Can you work these out from the model? Positions are in its coordinate system, mm. Give positions to 0.01 mm unless a question says otherwise; leave off trailing zeros.
```python
from build123d import *

# Parameters (mm, degrees)
BOSS_EXTRUDE1_DEPTH = 2
SKETCH2_R           = 1.42
CUT_EXTRUDE2_DEPTH  = 6.35


with BuildPart() as part:
    # Sketch1 → Boss-Extrude1 (new body)
    with BuildSketch(Plane(origin=(0, 0, 0), x_dir=(1, 0, 0), z_dir=(0, 1, 0))):
        with BuildLine():
            Line((-82.5, 25), (-82.5, -15.475))
            ThreePointArc((-82.5, -15.475), (-79.710192091, -22.210192091), (-72.975, -25))
            Line((-72.975, -25), (82.5, -25))
            Line((82.5, -25), (82.5, 25))
            Line((82.5, 25), (-82.5, 25))
        make_face()
    extrude(amount=BOSS_EXTRUDE1_DEPTH)

    # Sketch2 → Cut-Extrude2 (cut)
    with BuildSketch(Plane(origin=(0, 2, 0), x_dir=(1, 0, 0), z_dir=(0, 1, 0))):
        with BuildLine():
            ThreePointArc((-68.045, -15.475), (-66.625, -16.895), (-65.205, -15.475))
            Line((-65.205, -15.475), (-68.045, -15.475))
        make_face()
        with BuildLine():
            Line((-68.045, -15.475), (-65.205, -15.475))
            ThreePointArc((-65.205, -15.475), (-66.625, -14.055), (-68.045, -15.475))
        make_face()
        with Locations(Location((-72.975, -9.125, 0), (0, 0, 270))):
            Circle(SKETCH2_R)
        with BuildLine():
            ThreePointArc((-77.905, -15.475), (-79.325, -14.055), (-80.745, -15.475))
            Line((-80.745, -15.475), (-77.905, -15.475))
        make_face()
        with BuildLine():
            Line((-77.905, -15.475), (-80.745, -15.475))
            ThreePointArc((-80.745, -15.475), (-79.325, -16.895), (-77.905, -15.475))
        make_face()
        with Locations(Location((-72.975, -21.825, 0), (0, 0, 270))):
            Circle(SKETCH2_R)
        with BuildLine():
            ThreePointArc((-75.475, -15.475), (-72.975, -17.975), (-70.475, -15.475))
            Line((-70.475, -15.475), (-75.475, -15.475))
        make_face()
        with BuildLine():
            Line((-75.475, -15.475), (-70.475, -15.475))
            ThreePointArc((-70.475, -15.475), (-72.975, -12.975), (-75.475, -15.475))
        make_face()
    extrude(amount=-CUT_EXTRUDE2_DEPTH, mode=Mode.SUBTRACT)


solid = part.part
```
1) Please list where these lines run through material, in increasing order: L1, parallel to Z at x = -72, y = 0.2; L2, parallel to X at y = 1.75, z = 22; L3, parallel to Z at x = -66, y = 1.3.
Values follow:
L1: z = -25 to 8.09, 10.16 to 13.17, 17.78 to 20.79, 22.86 to 25
L2: x = -79.91 to -74.38, -71.57 to 82.5
L3: z = -25 to 14.2, 16.75 to 25
2) If we mould it in two halves opening along Z, with no side actions, what happens to faces 1 (the face through (-1, 0, 0)), 2 (the face through (-74.235, 1.014, 9.78)), 3 (the face through (-67.672, 1.014, 14.515)), 4 (the face through (-79.78, 0.99, 22.14))? For each: +Z half, -Z half, draft (parallel to the pull), parting line (faces both ways), or undercut.
Values follow:
face 1: draft
face 2: undercut
face 3: undercut
face 4: +Z half
3) For pin 1 Ø4.5 at (x, z) = (-66.625, 15.475) entering from +Y, with a flat end and sliding along its axis, tell me the tip position at first contact or that it passes through.
Values follow:
pin 1: stops at y = 2
